For this review, take the finished solid that the model builds, in its own axes (mm). Face numbers are marked on the shaded views. A direction names the side the tool comes from. Round coordinates to 2 decimals unless told otherwise and drop trailing zeros. Order: outer loops, then holes, each group sorted by start corner. A loop starts at its lowest first (then second) coordinate and runs counter-clockwise, first axis right, second up. Notation, with made-up numbers: (-7, 48.25) - (18, 48.25) arc R13 ccw to (18, 54.25) - close; hole circle Ø11 at (-33, 56). An arc over 180 degrees is marked (long way). One line per item, written item: value.
Autodesk Inventor part; units mm, degrees
ref_plane "WorkPlane2" through (0, 0, 0) normal (0, 0, 1) x (1, 0, 0)
ref_plane "Work Plane2" through (0, 0, -2.35) normal (0, 0, 1) x (1, 0, 0)
ref_plane "WorkPlane3" through (0, 0, 7) normal (0, 0, 1) x (1, 0, 0)
ref_plane "WorkPlane2" through (0, 0, 0) normal (0, 0, 1) x (1, 0, 0)
sketch "Sketch1" plane through (0, 0, 0) normal (1, 0, 0) x (0, 1, 0)
  point P0 (0, 0)
ref_plane "Work Plane2" through (0, 0, -2.35) normal (0, 0, 1) x (1, 0, 0)
ref_plane "WorkPlane3" through (0, 0, 7) normal (0, 0, 1) x (1, 0, 0)
sketch "Sketch2" plane through (0, 0, 0) normal (0, 1, 0) x (-1, 0, 0)
  point P0 (0, 0)
sketch "Sketch3" plane through (0, 0, 0) normal (1, 0, 0) x (0, 1, 0)
  line L0 (1.5, -3.35) -> (1.25, -2.85)
  line L1 (1.5, -20.7) -> (1.5, -3.35)
  line L2 (0, -20.7) -> (1.5, -20.7)
  line L3 (0, 0) -> (0, -20.7)
  arc A0 (2.75, -0.7) -> (0, 0) centre (0, -5.7518) ccw
  line L4 (2.75, -0.85) -> (2.75, -0.7)
  line L5 (1.25, -2.35) -> (2.75, -0.85)
  line L6 (1.25, -2.85) -> (1.25, -2.35)
  line L7 (0, -31.6445) -> (0, 31.6445) construction
  line L8 (0, -31.6445) -> (0, 31.6445)
  line L9 (0, -44.3023) -> (0, 44.3023)
  dimension "d2" = 1.5
  dimension "d4" = 1.25
  dimension "d6" = 0.5
  dimension "d8" = 1.65
  dimension "d10" = 135
  dimension "d12" = 2.75
  dimension "d14" = 0
  dimension "d16" = 0.7
  dimension "d18" = 20
  dimension "d22" = 17.35
revolve "Revolution1" add sketch "Sketch3" angle 360 about axis through (0, 0, -31.6445) along (0, 0, 1)
fillet "Fillet1" radius 0.8 1 edges at (0, -1.25, -2.35)
sketch "Sketch4" plane through (0, 0, 0) normal (0, 1, 0) x (-1, 0, 0)
  line L0 (0, 0) -> (-1.7, 0)
  line L1 (0, -1.4167) -> (0, 0)
  line L2 (-1.7, 0) -> (-0.2833, -1.4167)
  line L3 (0, -6.9021) -> (0, 1.1504)
  arc A0 (2.75, -0.7) -> (-2.75, -0.7) centre (0, -5.7518) ccw
  line L4 (0, -1.4167) -> (-0.2833, -1.4167)
  point P0 (0, -1.7)
  dimension "d30" = 45
  dimension "d33" = 3.4
  dimension "d34" = 0.2833
  dimension "d35" = 90
extrude "Extrusion1" cut sketch "Sketch4" along normal mid plane 0.5667
pattern_circular "PolarArray1" count 4 over 360 about axis through (0, 0, -10) along (0, 0, 1) of "Extrusion1"
thread "Thread1"
ref_plane "MSC_PF1" through (0, 0, 0) normal (1, 0, 0) x (0, 1, 0)
ref_plane "MSC_PT1" through (0, 2.75, -0.85) normal (0, 0, -1) x (-1, 0, 0)
equation "\"d2\" = 0.5 * NND"
equation "\"d4\" = 0.5 * msp_mdtds"
equation "\"d6\" = msp_x"
equation "\"d8\" = ParK"
equation "\"d12\" = 0.5 * Dk"
equation "\"d16\" = ParF"
equation "\"d18\" = NLG"
equation "\"d22\" = b"
equation "\"d24\" = r"
equation "\"d33\" = M"
equation "\"d31\" = 0.166667 * M"
equation "\"d39\" = b"
equation "\"PTC\" = 0.5"
equation "\"msp_x\" = PTC"
equation "\"NLG\" = 20"
equation "\"NND\" = 3"
equation "\"ParK\" = 1.65"
equation "\"r\" = 0.8"
equation "\"msp_mdtds\" = NND - PTC"
equation "\"b\" = 17.35"
equation "\"Dk\" = 5.5"
equation "\"ParF\" = 0.7"
equation "\"M\" = 3.4"
equation "\"ParA\" = 1"
equation "\"THREADDIA\" = NND"
equation "\"TEMPLATE\" = 1.2345"
properties part number "ISO 7047 - M3x20 - 4.8 - H" material "Steel"
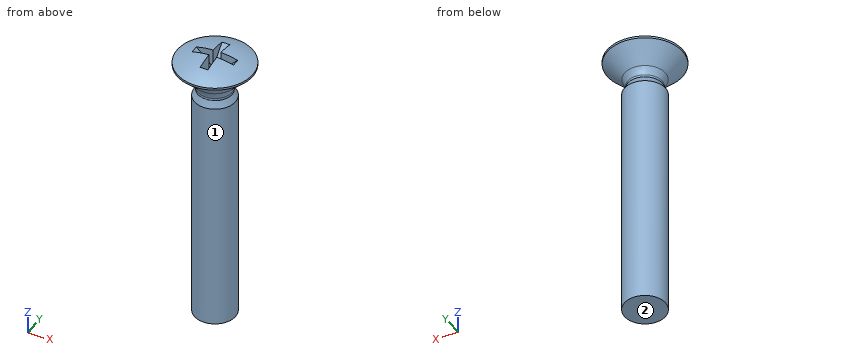
Item 1: For P1, Ø3, axis at y = 0, z = -18, coming from the +X side; P2, Ø1.5, axis at x = 0, z = -11.5, coming from the +Y side; P3, Ø1.3, axis at y = -1, z = -0.5, coming from the -X side, all flat-tipped, find the tip position at first contact; note any pin that passes through.
Returned:
P1: x = 1.5
P2: y = 1.5
P3: x = -2.72
Item 2: Take a section at A-A (z = -5.5). Write out the cut boundary in (x, y).
Returned:
outline: circle Ø3 at (0, 0)
Item 3: Wall thickness on line 1 (Y direction, x = -0.2, z = -6); line 2 (Y direction, x = 0, z = -1.25); line 3 (Z direction, x = -2.4, y = -0.7): over which ranges is each line inside the solid? List them lowest first.
Returned:
line 1: -1.49 to 1.49
line 2: -2.35 to -0.45, 0.45 to 2.35
line 3: -1.1 to -0.57
Item 4: Machinability: for the marked faces 1 and 2, which of the approach directions +Z, -Z, +X, -X, +Y, -Y give a long, thin tool a straight path to every point of the face, cutting with its end or side? Answer none if there is none.
Returned:
face 1: -Z
face 2: -Z, +X, -X, +Y, -Y
